Here's how the part is built. I have some questions about the finished solid (model axes, mm). A direction names the side the tool comes from. Round coordinates to 2 decimals unless told otherwise and drop trailing zeros. Loops run counter-clockwise (first coordinate to the right, second up) from the corner with the lowest first, then second, coordinate; pieces in that order, holes last. Notation, with made-up numbers: M 27.5,-11 L 79.5,-11 A34 ccw 79.5,22 Z; hole C 54.5,43 d6. An arc over 180 degrees is marked long. Answer as a JSON object with one key per item and string values.
from build123d import *

# Parameters (mm, degrees)
F0_W     = 228.6
F0_H     = 152.4
F1_DEPTH = 76.2
F3_DEPTH = 152.401
F5_DEPTH = 76.2


with BuildPart() as f1:
    # F0 (on Front) → F1 (new body, symmetric)
    with BuildSketch(Plane.XZ):
        Rectangle(F0_W, F0_H)
    extrude(amount=F1_DEPTH, both=True)

    # F2 (on face) → F3 (cut, through all)
    with BuildSketch(Plane(origin=(0, 76.2, 0), x_dir=(-1, 0, 0), z_dir=(0, 1, 0))):
        Polygon((-114.3, 0), (-12.709387, 76.2), (-114.3, 76.2), align=None)
    extrude(amount=-F3_DEPTH, mode=Mode.SUBTRACT)

    # F4 (on face) → F5 (cut)
    with BuildSketch(Plane(origin=(0, 76.2, 0), x_dir=(-1, 0, 0), z_dir=(0, 1, 0))):
        Polygon((-12.709387, 0), (-12.709387, 76.2), (-114.3, 0), align=None)
    extrude(amount=-F5_DEPTH, mode=Mode.SUBTRACT)


solid = f1.part
Item 1: I want a section at C-C on y = -40. List the corners of the cut face in (x, z) for me, plus the area to 3 significant figures.
Solution:
{"outline": "M -114.3,-76.2 L 114.3,-76.2 L 114.3,0 L 12.71,76.2 L -114.3,76.2 Z", "area": "31,000 mm2"}
Item 2: I want a section at A-A on y = 8. List the corners of the cut face in (x, z) for me, plus the area to 3 significant figures.
Solution:
{"outline": "M -114.3,-76.2 L 114.3,-76.2 L 114.3,0 L 12.71,0 L 12.71,76.2 L -114.3,76.2 Z", "area": "27,100 mm2"}
Item 3: I want a section at B-B on z = 30. List the corners of the cut face in (x, y) for me, plus the area to 3 significant figures.
Solution:
{"outline": "M -114.3,-76.2 L 74.3,-76.2 L 74.3,0 L 12.71,0 L 12.71,76.2 L -114.3,76.2 Z", "area": "24,000 mm2"}
Item 4: For P1, Ø1.5, axis at y = 11.5, z = 51, coming from the +X side; P2, Ø3, axis at x = 45, y = -51, coming from the +Z side, each with a flat end and sliding along its axis, tell me the tip position at first contact or that it passes through.
Solution:
{"P1": "stops at x = 12.71", "P2": "stops at z = 53.1"}
Item 5: If I drill on L1, parallel to X at y = 5, z = 9; L2, parallel to Y at x = 18, z = 54; L3, parallel to X at y = -43, z = 29, over which ranges is the centre line in solid material (lowest first)? Write a range as from..to.
Solution:
{"L1": "x = -114.3..12.71", "L2": "y = -76.2..0", "L3": "x = -114.3..75.64"}
Item 6: For faces 1 (the face through (64, 39, 0)), 2 (the face through (64.216, -37.567, 37.567)), which set-ups out of +Z, -Z, +X, -X, +Y, -Y let a thin tool reach every point of the face, with its end or its side?
Solution:
{"face 1": "+Z, +X, +Y", "face 2": "+Z, +X, +Y, -Y"}
